Here's how the part is built. I have some questions about the finished solid (model axes, mm). Coordinates: 2 decimals unless noted, no trailing zeros. Write each loop counter-clockwise with the first axis right and the second up, starting at its lowest first coordinate (ties: lowest second). Pieces come first, ordered by that corner, then holes. Notation, with made-up numbers: M 71,52.25 L 106,52.25 A9 cw 106,64.25 Z; hole C -1.75,-25 d10. An arc over 180 degrees is marked long. Use a Markdown table: item, result.
```python
from build123d import *

# Parameters (mm, degrees)
CYLINDER128_R                                = 2
CYLINDER128_DEPTH                            = 10
CYLINDER128_PITCH_ANGLE                      = 90
CYLINDER131_R                                = 2
CYLINDER131_DEPTH                            = 10
CYLINDER131_PITCH_ANGLE                      = 90
CYLINDER130_R                                = 2
CYLINDER130_DEPTH                            = 10
CYLINDER130_PITCH_ANGLE                      = 90
CYLINDER129_R                                = 2
CYLINDER129_DEPTH                            = 10
CYLINDER129_PITCH_ANGLE                      = 90
CYLINDER127_R                                = 7.5
CYLINDER127_DEPTH                            = 10
CYLINDER127_PITCH_ANGLE                      = 90
CYLINDER125_R                                = 3.25
CYLINDER125_DEPTH                            = 10
CYLINDER125_PITCH_ANGLE                      = 90
CYLINDER126_R                                = 3.25
CYLINDER126_DEPTH                            = 10
CYLINDER126_PITCH_ANGLE                      = 90
CYLINDER124_R                                = 4
CYLINDER124_DEPTH                            = 10
CYLINDER124_PITCH_ANGLE                      = 90
RECTANGLE159_W                               = 7.5
RECTANGLE159_H                               = 3
EXTRUDE205_DEPTH                             = 3
RECTANGLE155_W                               = 3
RECTANGLE155_H                               = 7.5
EXTRUDE204_DEPTH                             = 3
RECTANGLE140_W                               = 17.5
RECTANGLE140_H                               = 3
EXTRUDE181_DEPTH                             = 3
RECTANGLE142_W                               = 17.5
RECTANGLE142_H                               = 3
EXTRUDE183_DEPTH                             = 3
RECTANGLE141_W                               = 17.5
RECTANGLE141_H                               = 3
EXTRUDE182_DEPTH                             = 3
RECTANGLE139_W                               = 17.5
RECTANGLE139_H                               = 3
EXTRUDE180_DEPTH                             = 3
RECTANGLE129_AS_DRAWN_W                      = 25
RECTANGLE129_AS_DRAWN_H                      = 3
EXTRUDE172_DEPTH                             = 3
EXTRUDE172_ONTO_RECTANGLE129_ROLL_ANGLE      = -90
EXTRUDE172_ONTO_RECTANGLE129_PLACEMENT_ANGLE = 180
RECTANGLE132_AS_DRAWN_W                      = 3
RECTANGLE132_AS_DRAWN_H                      = 19.5
EXTRUDE169_DEPTH                             = 3
EXTRUDE169_ONTO_RECTANGLE132_ROLL_ANGLE      = -90
EXTRUDE169_ONTO_RECTANGLE132_PLACEMENT_ANGLE = 180
BOX012_W                                     = 3
BOX012_H                                     = 155
BOX012_DEPTH                                 = 210


with BuildPart() as cylinder159:
    # Cylinder128 → Cylinder128 (new body)
    with BuildSketch(Plane.XY):
        Circle(CYLINDER128_R)
    extrude(amount=CYLINDER128_DEPTH)


with BuildPart() as cylinder159_1:
    # Cylinder128 pitch: moved
    add(cylinder159.part.rotate(Axis((0, 0, 0), (0, 1, 0)), CYLINDER128_PITCH_ANGLE))


with BuildPart() as cylinder159_2:
    # Cylinder128 placement: moved
    add(cylinder159_1.part.moved(Location((-173, 44, 81.5))))


with BuildPart() as cylinder162:
    # Cylinder131 → Cylinder131 (new body)
    with BuildSketch(Plane.XY):
        Circle(CYLINDER131_R)
    extrude(amount=CYLINDER131_DEPTH)


with BuildPart() as cylinder162_1:
    # Cylinder131 pitch: moved
    add(cylinder162.part.rotate(Axis((0, 0, 0), (0, 1, 0)), CYLINDER131_PITCH_ANGLE))


with BuildPart() as cylinder162_2:
    # Cylinder131 placement: moved
    add(cylinder162_1.part.moved(Location((-173, 32.5, 70))))


with BuildPart() as cylinder161:
    # Cylinder130 → Cylinder130 (new body)
    with BuildSketch(Plane.XY):
        Circle(CYLINDER130_R)
    extrude(amount=CYLINDER130_DEPTH)


with BuildPart() as cylinder161_1:
    # Cylinder130 pitch: moved
    add(cylinder161.part.rotate(Axis((0, 0, 0), (0, 1, 0)), CYLINDER130_PITCH_ANGLE))


with BuildPart() as cylinder161_2:
    # Cylinder130 placement: moved
    add(cylinder161_1.part.moved(Location((-173, 55.5, 70))))


with BuildPart() as cylinder160:
    # Cylinder129 → Cylinder129 (new body)
    with BuildSketch(Plane.XY):
        Circle(CYLINDER129_R)
    extrude(amount=CYLINDER129_DEPTH)


with BuildPart() as cylinder160_1:
    # Cylinder129 pitch: moved
    add(cylinder160.part.rotate(Axis((0, 0, 0), (0, 1, 0)), CYLINDER129_PITCH_ANGLE))


with BuildPart() as cylinder160_2:
    # Cylinder129 placement: moved
    add(cylinder160_1.part.moved(Location((-173, 44, 58.5))))


with BuildPart() as fusion064062:
    # Cylinder127 → Cylinder127 (new body)
    with BuildSketch(Plane.XY):
        Circle(CYLINDER127_R)
    extrude(amount=CYLINDER127_DEPTH)


with BuildPart() as fusion064062_1:
    # Cylinder127 pitch: moved
    add(fusion064062.part.rotate(Axis((0, 0, 0), (0, 1, 0)), CYLINDER127_PITCH_ANGLE))


with BuildPart() as fusion064062_2:
    # Cylinder127 placement: moved
    add(fusion064062_1.part.moved(Location((-175, 44, 70))))

    # Fusion064062: union Cylinder159, Cylinder162, Cylinder161, Cylinder160
    add(cylinder159_2.part)
    add(cylinder162_2.part)
    add(cylinder161_2.part)
    add(cylinder160_2.part)


with BuildPart() as cylinder156:
    # Cylinder125 → Cylinder125 (new body)
    with BuildSketch(Plane.XY):
        Circle(CYLINDER125_R)
    extrude(amount=CYLINDER125_DEPTH)


with BuildPart() as cylinder156_1:
    # Cylinder125 pitch: moved
    add(cylinder156.part.rotate(Axis((0, 0, 0), (0, 1, 0)), CYLINDER125_PITCH_ANGLE))


with BuildPart() as cylinder156_2:
    # Cylinder125 placement: moved
    add(cylinder156_1.part.moved(Location((-172, -30, 70))))


with BuildPart() as cylinder157:
    # Cylinder126 → Cylinder126 (new body)
    with BuildSketch(Plane.XY):
        Circle(CYLINDER126_R)
    extrude(amount=CYLINDER126_DEPTH)


with BuildPart() as cylinder157_1:
    # Cylinder126 pitch: moved
    add(cylinder157.part.rotate(Axis((0, 0, 0), (0, 1, 0)), CYLINDER126_PITCH_ANGLE))


with BuildPart() as cylinder157_2:
    # Cylinder126 placement: moved
    add(cylinder157_1.part.moved(Location((-172, -58, 70))))


with BuildPart() as fusion064063:
    # Cylinder124 → Cylinder124 (new body)
    with BuildSketch(Plane.XY):
        Circle(CYLINDER124_R)
    extrude(amount=CYLINDER124_DEPTH)


with BuildPart() as fusion064063_1:
    # Cylinder124 pitch: moved
    add(fusion064063.part.rotate(Axis((0, 0, 0), (0, 1, 0)), CYLINDER124_PITCH_ANGLE))


with BuildPart() as fusion064063_2:
    # Cylinder124 placement: moved
    add(fusion064063_1.part.moved(Location((-173, -44, 70))))

    # Fusion064060: union Cylinder156, Cylinder157
    add(cylinder156_2.part)
    add(cylinder157_2.part)

    # Fusion064063: union Fusion064062
    add(fusion064062_2.part)


with BuildPart() as extrude205:
    # Rectangle159 → Extrude205 (new body)
    with BuildSketch(Plane(origin=(-169, 70.5, 95), x_dir=(0, -1, 0), z_dir=(-1, 0, 0))):
        with Locations((3.75, -1.5)):
            Rectangle(RECTANGLE159_W, RECTANGLE159_H)
    extrude(amount=-EXTRUDE205_DEPTH)


with BuildPart() as fusion064057:
    # Rectangle155 → Extrude204 (new body)
    with BuildSketch(Plane(origin=(-169, 75, 80), x_dir=(0, -1, 0), z_dir=(-1, 0, 0))):
        with Locations((-1.5, 3.75)):
            Rectangle(RECTANGLE155_W, RECTANGLE155_H)
    extrude(amount=-EXTRUDE204_DEPTH)

    # Fusion064057: union Extrude205
    add(extrude205.part)


with BuildPart() as extrude181:
    # Rectangle140 → Extrude181 (new body)
    with BuildSketch(Plane(origin=(114, 20.5, -70), x_dir=(0, 1, 0), z_dir=(1, 0, 0))):
        with Locations((8.75, -1.5)):
            Rectangle(RECTANGLE140_W, RECTANGLE140_H)
    extrude(amount=-EXTRUDE181_DEPTH)


with BuildPart() as extrude183:
    # Rectangle142 → Extrude183 (new body)
    with BuildSketch(Plane(origin=(114, -37, -112), x_dir=(0, 1, 0), z_dir=(1, 0, 0))):
        with Locations((8.75, -1.5)):
            Rectangle(RECTANGLE142_W, RECTANGLE142_H)
    extrude(amount=-EXTRUDE183_DEPTH)


with BuildPart() as extrude182:
    # Rectangle141 → Extrude182 (new body)
    with BuildSketch(Plane(origin=(114, 20.5, -112), x_dir=(0, 1, 0), z_dir=(1, 0, 0))):
        with Locations((8.75, -1.5)):
            Rectangle(RECTANGLE141_W, RECTANGLE141_H)
    extrude(amount=-EXTRUDE182_DEPTH)


with BuildPart() as fusion064045:
    # Rectangle139 → Extrude180 (new body)
    with BuildSketch(Plane(origin=(114, -37, -70), x_dir=(0, 1, 0), z_dir=(1, 0, 0))):
        with Locations((8.75, -1.5)):
            Rectangle(RECTANGLE139_W, RECTANGLE139_H)
    extrude(amount=-EXTRUDE180_DEPTH)

    # Fusion064045: union Extrude181, Extrude183, Extrude182
    add(extrude181.part)
    add(extrude183.part)
    add(extrude182.part)


with BuildPart() as fusion064045_1:
    # Fusion064045 placement: moved
    add(fusion064045.part.moved(Location((-280, 0, 0))))


with BuildPart() as extrude172:
    # Rectangle129 as drawn → Extrude172 (new)
    with BuildSketch(Plane.XY):
        with Locations((12.5, 1.5)):
            Rectangle(RECTANGLE129_AS_DRAWN_W, RECTANGLE129_AS_DRAWN_H)
    extrude(amount=-EXTRUDE172_DEPTH)


with BuildPart() as extrude172_1:
    # Extrude172 onto Rectangle129 roll: moved
    add(extrude172.part.rotate(Axis((0, 0, 0), (1, 0, 0)), EXTRUDE172_ONTO_RECTANGLE129_ROLL_ANGLE))


with BuildPart() as extrude172_2:
    # Extrude172 onto Rectangle129 placement: moved
    add(extrude172_1.part.moved(Location((64, -77, -70))).rotate(Axis((64, -77, -70), (0, 0, 1)), EXTRUDE172_ONTO_RECTANGLE129_PLACEMENT_ANGLE))


with BuildPart() as extrude172_3:
    # Extrude172 placement: moved
    add(extrude172_2.part.moved(Location((-208, 0, 0))))


with BuildPart() as extrude169:
    # Rectangle132 as drawn → Extrude169 (new)
    with BuildSketch(Plane.XY):
        with Locations((1.5, 9.75)):
            Rectangle(RECTANGLE132_AS_DRAWN_W, RECTANGLE132_AS_DRAWN_H)
    extrude(amount=-EXTRUDE169_DEPTH)


with BuildPart() as extrude169_1:
    # Extrude169 onto Rectangle132 roll: moved
    add(extrude169.part.rotate(Axis((0, 0, 0), (1, 0, 0)), EXTRUDE169_ONTO_RECTANGLE132_ROLL_ANGLE))


with BuildPart() as extrude169_2:
    # Extrude169 onto Rectangle132 placement: moved
    add(extrude169_1.part.moved(Location((114, -77, -92.5))).rotate(Axis((114, -77, -92.5), (0, 0, 1)), EXTRUDE169_ONTO_RECTANGLE132_PLACEMENT_ANGLE))


with BuildPart() as extrude169_3:
    # Extrude169 placement: moved
    add(extrude169_2.part.moved(Location((-280, 0, 0))))


with BuildPart() as fusion064037:
    # Fusion064037 base: copy of Extrude169
    add(extrude169_3.part)

    # Fusion064037: union Extrude172
    add(extrude172_3.part)


with BuildPart() as fusion064037_1:
    # Fusion064037 placement: moved
    add(fusion064037.part.moved(Location((0, 152, 0))))


with BuildPart() as fusion064031:
    # Fusion064031 base: copy of Extrude169
    add(extrude169_3.part)

    # Fusion064031: union Extrude172
    add(extrude172_3.part)


with BuildPart() as cut035053:
    # Box012 → Box012 (new body)
    with BuildSketch(Plane(origin=(-169, -77, -115), x_dir=(1, 0, 0), z_dir=(0, 0, 1))):
        with Locations((1.5, 77.5)):
            Rectangle(BOX012_W, BOX012_H)
    extrude(amount=BOX012_DEPTH)

    # Cut035021: cut Fusion064031
    add(fusion064031.part, mode=Mode.SUBTRACT)

    # Cut035024: cut Fusion064037
    add(fusion064037_1.part, mode=Mode.SUBTRACT)

    # Cut035032: cut Fusion064045
    add(fusion064045_1.part, mode=Mode.SUBTRACT)

    # Cut035042: cut Fusion064057
    add(fusion064057.part, mode=Mode.SUBTRACT)

    # Cut035053: cut Fusion064063
    add(fusion064063_2.part, mode=Mode.SUBTRACT)


solid = cut035053.part
```
1. Will these pins go through, and if not, where does the flat tip stop? pin 1 Ø5 at (y, z) = (-58, 70) entering from +X; pin 2 Ø1.5 at (x, z) = (-167.5, -104) entering from +Y.
Answers follow:
| item | result |
|---|---|
| pin 1 | passes through |
| pin 2 | stops at y = 75 |
2. Suppose I cut it at A-A on y = -30. Write out the boundary of the cut face in (x, z).
Answers follow:
| item | result |
|---|---|
| outline | M -169,-112 L -166,-112 L -166,-73 L -169,-73 Z; M -169,-70 L -166,-70 L -166,66.75 L -169,66.75 Z; M -169,73.25 L -166,73.25 L -166,95 L -169,95 Z |
3. I need wall thicknesses on probe 1 along Z at (x, y) = (-166.95, 44); probe 2 along Z at (x, y) = (-167.1, 32.5); probe 3 along Z at (x, y) = (-166.95, -30). Which ranges of each line are inside material? Lowest first, please.
Answers follow:
| item | result |
|---|---|
| probe 1 | z = -115 to 56.5, 60.5 to 62.5, 77.5 to 79.5, 83.5 to 95 |
| probe 2 | z = -112 to -73, -70 to 68, 72 to 95 |
| probe 3 | z = -112 to -73, -70 to 66.75, 73.25 to 95 |
4. Suppose I cut it at B-B on y = -58. Write out the boundary of the cut face in (x, z), and give its area (4 significant figures).
Answers follow:
| item | result |
|---|---|
| outline | M -169,-115 L -166,-115 L -166,66.75 L -169,66.75 Z; M -169,73.25 L -166,73.25 L -166,95 L -169,95 Z |
| area | 610.5 mm2 |
5. We'd pull the mould along Y, two halves only. Please class faces 1 (the face through (-169, -1, -11)), 2 (the face through (-167.521, 42.226, 57.577)): +Y half, -Y half, draft (parallel to the pull), parting line (faces both ways), or undercut.
Answers follow:
| item | result |
|---|---|
| face 1 | draft |
| face 2 | undercut |
6. Suppose I cut it at C-C on x = -166.6. State how many separate pieces and enclosed holes the cut face has, and give its area (3 significant figures).
Answers follow:
| item | result |
|---|---|
| separate pieces | 1 |
| enclosed holes | 10 |
| area | 31,800 mm2 |
